```python
from build123d import *

# Parameters (mm, degrees)
SKETCH1_R           = 3.175
BOSS_EXTRUDE1_DEPTH = 88.9
CUT_EXTRUDE1_DEPTH  = 210.541455785
CUT_EXTRUDE2_DEPTH  = 83.82
CUT_EXTRUDE3_DEPTH  = 82.661206718
BOSS_EXTRUDE2_DEPTH = 5.865878735
SKETCH6_W           = 7.62
SKETCH6_H           = 7.62
SKETCH6_R           = 3.175
BOSS_EXTRUDE3_DEPTH = 88.9


with BuildPart() as part:
    # Sketch1 → Boss-Extrude1 (new body)
    with BuildSketch(Plane.XY):
        with BuildLine():
            Line((-38.875279998, 168.243550653), (48.865926721, 168.243550653))
            Line((48.865926721, 168.243550653), (48.865926721, 53.943550653))
            Line((48.865926721, 53.943550653), (2.740491947, -36.582712205))
            ThreePointArc((2.740491947, -36.582712205), (-55.650204571, -55.55499958), (-74.622491947, 2.835696938))
            Line((-74.622491947, 2.835696938), (-38.875279998, 72.993550653))
            Line((-38.875279998, 72.993550653), (-38.875279998, 168.243550653))
        make_face()
        with Locations((-23.07761236, 59.263499889)):
            Circle(SKETCH1_R, mode=Mode.SUBTRACT)
        with Locations((22.13438764, 59.263499889)):
            Circle(SKETCH1_R, mode=Mode.SUBTRACT)
        with BuildLine():
            Line((-7.651542857, -31.287706), (15.41117453, 13.975425429))
            Line((15.41117453, 13.975425429), (-46.933419103, 31.488039305))
            Line((-46.933419103, 31.488039305), (-64.230457143, -2.459309266))
            ThreePointArc((-64.230457143, -2.459309266), (-50.355198367, -45.162964776), (-7.651542857, -31.287706))
        make_face(mode=Mode.SUBTRACT)
    extrude(amount=BOSS_EXTRUDE1_DEPTH)

    # Sketch2 → Cut-Extrude1 (cut, through all)
    with BuildSketch(Plane.ZY.offset(38.875279998)):
        Polygon((0, 168.243550653), (88.9, 116.917111722), (88.9, 168.243550653), align=None)
    extrude(amount=-CUT_EXTRUDE1_DEPTH, mode=Mode.SUBTRACT)

    # Sketch3 → Cut-Extrude2 (cut)
    with BuildSketch(Plane.XY.offset(88.9)):
        with BuildLine():
            Line((43.785926721, 111.837111722), (-33.795279998, 111.837111722))
            Line((-33.795279998, 111.837111722), (-33.795279998, 71.773950557))
            Line((-33.795279998, 71.773950557), (-70.096178804, 0.5294252))
            ThreePointArc((-70.096178804, 0.5294252), (-53.343932833, -51.028686437), (-1.785821196, -34.276440466))
            Line((-1.785821196, -34.276440466), (43.785926721, 55.163150749))
            Line((43.785926721, 55.163150749), (43.785926721, 111.837111722))
        make_face()
    extrude(amount=-CUT_EXTRUDE2_DEPTH, mode=Mode.SUBTRACT)

    # Sketch4 → Cut-Extrude3 (cut)
    with BuildSketch(Plane.ZY.offset(38.875279998)):
        Polygon((83.82, 78.073550653), (83.82, 113.984172354), (5.08, 159.44473255), (5.08, 78.073550653), align=None)
    extrude(amount=-CUT_EXTRUDE3_DEPTH, mode=Mode.SUBTRACT)

    # Sketch5 → Boss-Extrude2 (add, along a direction that is not the sketch's normal)
    with BuildSketch(Plane(origin=(0, 126.18266299, 72.851594444), x_dir=(1, 0, 0), z_dir=(0, 0.8660254037844417, 0.4999999999999947))):
        Polygon((-38.875279998, 84.121775326), (-74.887919552, 77.771775326), (-38.875279998, 71.421775326), align=None)
        Polygon((-38.875279998, 53.641775326), (-74.887919552, 47.291775326), (-38.875279998, 40.941775326), align=None)
        Polygon((-38.875279998, 24.648897465), (-74.887919552, 18.298897465), (-38.875279998, 11.948897465), align=None)
        Polygon((-38.875279998, -5.831102535), (-74.887919552, -12.181102535), (-38.875279998, -18.531102535), align=None)
    extrude(amount=-BOSS_EXTRUDE2_DEPTH, dir=(0, 1, 0))

    # Sketch6 → Boss-Extrude3 (add)
    # profile 1 of 2: a face of its own
    with BuildSketch(Plane.XY.offset(88.9)):
        with Locations((52.675926721, 113.107111722)):
            Rectangle(SKETCH6_W, SKETCH6_H)
        with Locations((52.675926721, 113.107111722)):
            Circle(SKETCH6_R, mode=Mode.SUBTRACT)
    # profile 2 of 2: a face of its own
    with BuildSketch(Plane.XY.offset(88.9)):
        Polygon((-62.514565319, 26.598840938), (-59.055157711, 33.388310653), (-65.844627425, 36.847718261), (-69.304035033, 30.058248546), align=None)
        with Locations((-64.179596372, 31.7232796)):
            Circle(SKETCH6_R, mode=Mode.SUBTRACT)
    extrude(amount=-BOSS_EXTRUDE3_DEPTH)


solid = part.part
```
The model under review builds one solid part; all positions refer to its coordinate system, in mm. A direction names the side the tool comes from. Round coordinates to 2 decimals unless told otherwise and drop trailing zeros. Order: outer loops, then holes, each group sorted by start corner. A loop starts at its lowest first (then second) coordinate and runs counter-clockwise, first axis right, second up. Notation, with made-up numbers: M 55,-12 L 62,-12 A21 ccw 62,2 Z; hole C -26.5,-6.75 d7. An arc over 180 degrees is marked long. Use a Markdown table: item, result.
1) Consider section A-A (y = 106). Write out the cut boundary in (x, z), then the cut area to 3 significant figures.
Report:
| item | result |
|---|---|
| outline | M -38.88,0 L 48.87,0 L 48.87,88.9 L 43.79,88.9 L 43.79,5.08 L -38.88,5.08 Z; M -38.88,83.82 L -33.8,83.82 L -33.8,88.9 L -38.88,88.9 Z |
| area | 897 mm^2 |
2) Tool access review of faces 1 (the face through (-54.09, -50.64, 47.58)), 2 (the face through (-3, 77, 5.08)), 3 (the face through (-15.325, 22.609, 2.504)): name each direction out of +Z, -Z, +X, -X, +Y, -Y from which nothing blocks a thin tool from reaching the whole face with its end or side.
Report:
| item | result |
|---|---|
| face 1 | +Z |
| face 2 | none |
| face 3 | +Z, -Z |
3) Consider section C-C (z = 74.5). Give the number of separate pieces and of enclosed holes in the cut face, then the cut area to 3 significant figures.
Report:
| item | result |
|---|---|
| separate pieces | 1 |
| enclosed holes | 2 |
| area | 2,490 mm^2 |
4) Consider section B-B (x = -14.5). Write out the cut boundary in (y, z).
Report:
| item | result |
|---|---|
| outline | M -54.62,0 L -40.29,0 L -40.29,5.08 L -48.65,5.08 L -48.65,88.9 L -54.62,88.9 Z; M 22.38,0 L 168.24,0 L 116.92,88.9 L 111.84,88.9 L 111.84,83.82 L 113.98,83.82 L 159.44,5.08 L 22.38,5.08 Z |
5) Insertion check: pin 1 (5 mm diameter, centred on y = 24.5, z = 13.5, fed in from -X); pin 2 (5.5 mm diameter, centred on x = 24, z = 86.5, fed in from -Y); pin 3 (1 mm diameter, centred on y = -33, z = 52, fed in from -X); pin 4 (5.5 mm diameter, centred on x = -23.08, y = 59.26, fed in from -Z). Each pin has a flat end and moves straight along its axis. Give the tip position at first contact, or say it passes through.
Report:
| item | result |
|---|---|
| pin 1 | x = -64.86 |
| pin 2 | y = -0.26 |
| pin 3 | x = -76.44 |
| pin 4 | through |
6) Consider section D-D (x = -52.5). Write out the cut boundary in (y, z).
Report:
| item | result |
|---|---|
| outline | M -57,0 L -43.96,0 L -43.96,5.08 L -51.45,5.08 L -51.45,88.9 L -57,88.9 Z; M 20.56,0 L 46.25,0 L 46.25,88.9 L 35.06,88.9 L 35.06,5.08 L 20.56,5.08 Z; M 112.25,86.82 L 116.2,79.98 L 122.07,79.98 L 118.12,86.82 Z; M 127.49,60.42 L 131.44,53.59 L 137.31,53.59 L 133.36,60.42 Z; M 141.99,35.31 L 145.94,28.48 L 151.8,28.48 L 147.85,35.31 Z; M 157.23,8.92 L 161.18,2.08 L 167.04,2.08 L 163.09,8.92 Z |
7) Wall thickness on line 1 along Y through (x, z) = (-37, 18.5); line 2 along Y through (x, z) = (-45, 35.5); line 3 along Y through (x, z) = (24, 81): over which ranges is each line inside the solid? List them lowest first. Write a range as [from, to].
Report:
| item | result |
|---|---|
| line 1 | [-60.27, -55.19], [65.48, 78.07], [151.7, 157.56] |
| line 2 | [-59.33, -54.12], [49.78, 60.97], [141.88, 147.75] |
| line 3 | [5.14, 16.33], [115.61, 121.48] |
8) Draft analysis for pull direction Y (two halves, no side actions). For faces 4 (the face through (-50.97, -44.84, 2.5)), 5 (the face through (-56.63, 148.546, 29.108)), 6 (the face through (23.84, 61.94, 2.5)), 7 (the face through (26.126, 9.314, 43.828)), state which applies: released by +Y, released by -Y, zero draft, split by the parting line, or undercut.
Report:
| item | result |
|---|---|
| face 4 | undercut |
| face 5 | zero draft |
| face 6 | undercut |
| face 7 | released by -Y |
